Verification items for this drawing (mm, ordinates from the low corner). A direction names the side the tool comes from. Give positions to 0.01 mm unless a question says otherwise; leave off trailing zeros. Order: outer loops, then holes, each group sorted by start corner. A loop starts at its lowest first (then second) coordinate and runs counter-clockwise, first axis right, second up. Notation, with made-up numbers: M 20,-35.5 L 31,-35.5 A9 cw 31,-23.5 Z; hole C 6.25,78.25 d6. An arc over 180 degrees is marked long. Answer as a JSON object with one key per item and string values.
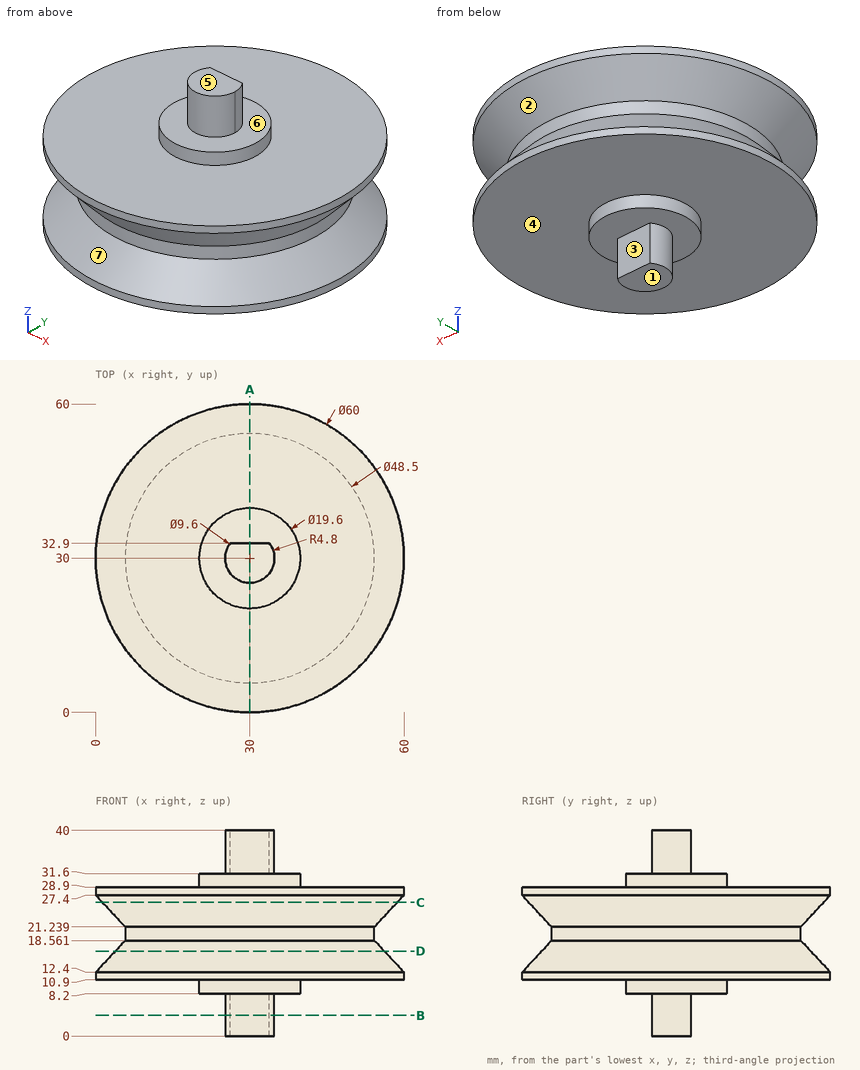
Q1. Material ranges on L1, parallel to Z at x = 11, y = 39; L2, parallel to Z at x = 16.5, y = 6.5 (1 decimal); L3, parallel to Z at x = 16, y = 50 (1 decimal), recorded low to high.
Resolved:
{"L1": "z = 10.9 to 28.9", "L2": "z = 10.9 to 15.5, 24.3 to 28.9", "L3": "z = 10.9 to 18.4, 21.4 to 28.9"}
Q2. Tool access check on the marked faces 4, 5, 6 and 7. Record the directions out of +Z, -Z, +X, -X, +Y, -Y that give a thin tool (end or side, any length) a straight path to the whole face; none if there is none.
Resolved:
{"face 4": "-Z", "face 5": "+Z, +X, -X, +Y, -Y", "face 6": "+Z", "face 7": "none"}
Q3. Section check C-C on z = 26. Record the cut outline in (x, y), then the cut area to 3 significant figures.
Resolved:
{"outline": "C 30,30 d57.39", "area": "2,590 mm²"}
Q4. Section check D-D on z = 16.5. Record the cut outline in (x, y).
Resolved:
{"outline": "C 30,30 d52.35"}
Q5. Release check for a two-part mould opening along Z. For the marked faces 1, 2 and 3 record: +Z half, -Z half, draft (parallel to the pull), parting line (faces both ways), or undercut.
Resolved:
{"face 1": "-Z half", "face 2": "undercut", "face 3": "draft"}
Q6. Section check A-A on x = 30. Record the cut outline in (y, z).
Resolved:
{"outline": "M 0,10.9 L 20.2,10.9 L 20.2,8.2 L 25.2,8.2 L 25.2,0 L 32.9,0 L 32.9,8.2 L 39.8,8.2 L 39.8,10.9 L 60,10.9 L 60,12.4 L 54.25,18.56 L 54.25,21.24 L 60,27.4 L 60,28.9 L 39.8,28.9 L 39.8,31.6 L 32.9,31.6 L 32.9,40 L 25.2,40 L 25.2,31.6 L 20.2,31.6 L 20.2,28.9 L 0,28.9 L 0,27.4 L 5.75,21.24 L 5.75,18.56 L 0,12.4 Z"}
Q7. Gauge pin test, flat ends, axial feed: pin 1 Ø10 at (x, y) = (26.5, 15) entering from -Z; pin 2 Ø1 at (x, z) = (27, 29) entering from -Y (1 decimal); pin 3 Ø12 at (y, z) = (19.5, 14.5) entering from +X. Record the tip position at first contact, or that the pin passes through.
Resolved:
{"pin 1": "stops at z = 10.9", "pin 2": "stops at y = 0.1", "pin 3": "stops at x = 59.6"}
Q8. Section check B-B on z = 4. Record the cut outline in (x, y) (1 decimal), then the cut area to 3 significant figures.
Resolved:
{"outline": "M 26.2,32.9 A4.8 ccw long 33.8,32.9 Z", "area": "62.2 mm²"}
